Can you work these out from the drawing? Everything is in mm from the part's minimum corner. A direction names the side the tool comes from. Coordinates: 2 decimals unless noted, no trailing zeros. Loops run counter-clockwise (first coordinate to the right, second up) from the corner with the lowest first, then second, coordinate; pieces in that order, holes last.
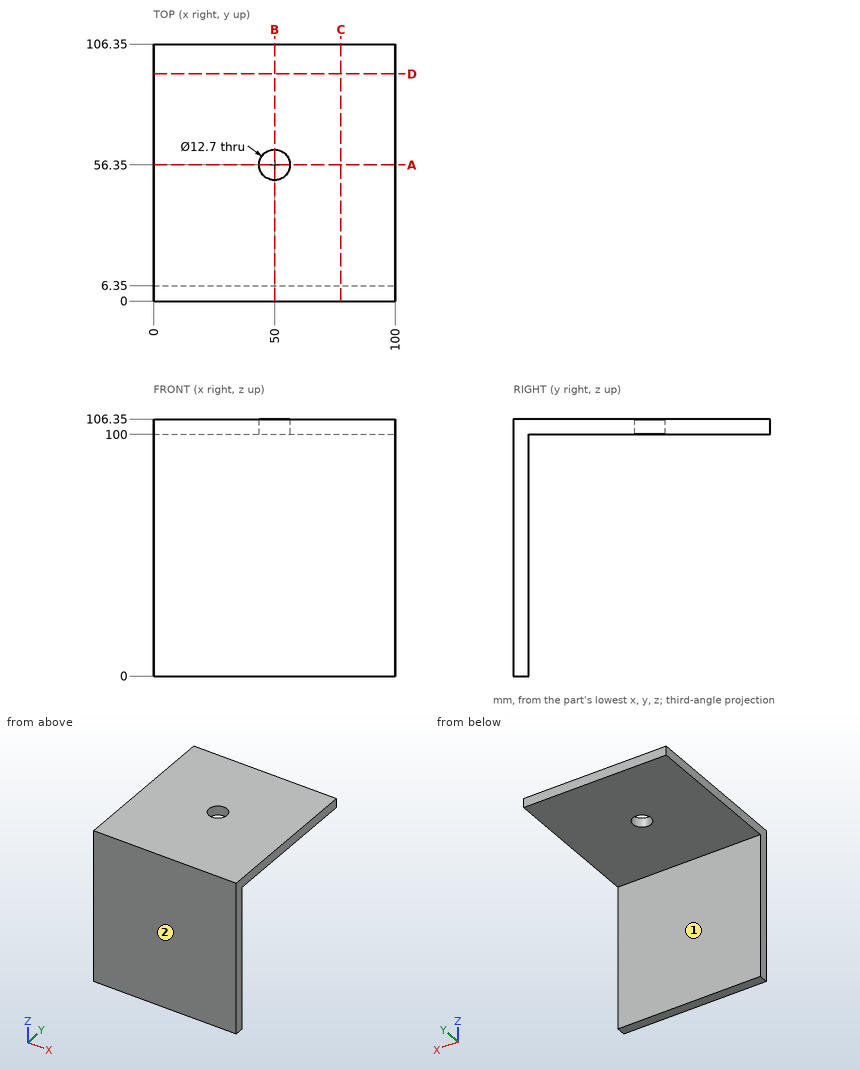
1) Imagine slicing it at D-D on y = 94. List the corners of the cut face in (x, z) for me, plus the area to 3 significant figures.
2) For the marked faces 1 and 2, which set-ups out of +Z, -Z, +X, -X, +Y, -Y let a thin tool reach every point of the face, with its end or its side?
3) Imagine slicing it at A-A on y = 56.35. List the corners of the cut face in (x, z) for me.
4) Imagine slicing it at C-C on x = 77.5. List the corners of the cut face in (y, z) for me.
5) Imagine slicing it at B-B on x = 50. List the corners of the cut face in (y, z) for me.
6) Will these pins go through, and if not, where does the flat tip stop? pin 1 (12 mm diameter, centred on x = 53, z = 68.5, fed in from +Y); pin 2 (16.5 mm diameter, centred on x = 50, y = 56.35, fed in from -Z).
7) If I drill on L1, parallel to Y at x = 50, z = 102; L2, parallel to X at y = 56, z = 104; L3, parallel to Y at x = 79.5, z = 83.5, over which ranges is the centre line in solid material (lowest first)?
Solved:
1. outline: (0, 100) - (100, 100) - (100, 106.35) - (0, 106.35) - close
1. area: 635 mm2
2. face 1: -Z, +X, -X, +Y
2. face 2: +Z, -Z, +X, -X, -Y
3. outline: (0, 100) - (43.65, 100) - (43.65, 106.35) - (0, 106.35) - close; (56.35, 100) - (100, 100) - (100, 106.35) - (56.35, 106.35) - close
4. outline: (0, 0) - (6.35, 0) - (6.35, 100) - (106.35, 100) - (106.35, 106.35) - (0, 106.35) - close
5. outline: (0, 0) - (6.35, 0) - (6.35, 100) - (50, 100) - (50, 106.35) - (0, 106.35) - close; (62.7, 100) - (106.35, 100) - (106.35, 106.35) - (62.7, 106.35) - close
6. pin 1: stops at y = 6.35
6. pin 2: stops at z = 100
7. L1: y = 0 to 50, 62.7 to 106.35
7. L2: x = 0 to 43.66, 56.34 to 100
7. L3: y = 0 to 6.35
